The listing builds one solid part. Answer for the finished solid, in the listing's coordinates (mm). Face numbers are marked on the shaded views. A direction names the side the tool comes from. Coordinates: 2 decimals unless noted, no trailing zeros. Order: outer loops, then holes, each group sorted by start corner. A loop starts at its lowest first (then second) coordinate and runs counter-clockwise, first axis right, second up. Notation, with made-up numbers: (72.25, 16) -> (109.25, 16) arc R9 ccw to (109.25, 27) -> close; hole circle Ø2 at (36, 46.5). An arc over 180 degrees is marked (long way). Write item = value, one per line.
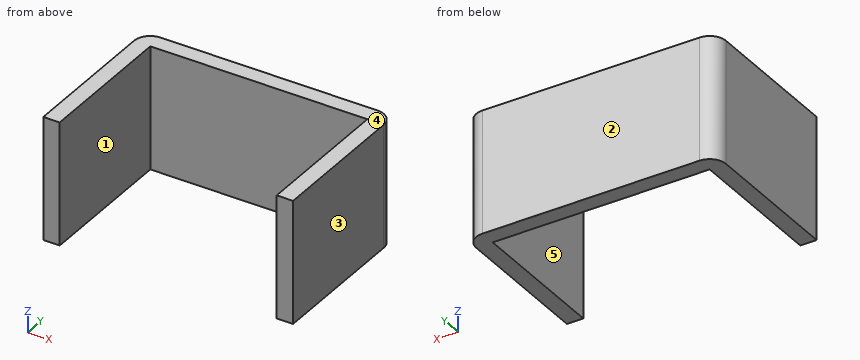
from build123d import *

# Parameters (mm, degrees)
BOSS_EXTRUDE1_DEPTH = 30


with BuildPart() as part:
    # Sketch1 → Boss-Extrude1 (new body)
    with BuildSketch(Plane.XY):
        with BuildLine():
            Line((0, 0), (0, 35))
            ThreePointArc((0, 35), (1.171572875, 37.828427125), (4, 39))
            Line((4, 39), (57, 39))
            ThreePointArc((57, 39), (59.828427125, 37.828427125), (61, 35))
            Line((61, 35), (61, 0))
            Line((61, 0), (57, 0))
            Line((57, 0), (57, 35))
            Line((57, 35), (4, 35))
            Line((4, 35), (4, 0))
            Line((4, 0), (0, 0))
        make_face()
    extrude(amount=BOSS_EXTRUDE1_DEPTH)


solid = part.part
Q1. Find the intervals of material crossed by line 1 along X through (y, z) = (11.5, 28.25); line 2 along Y through (x, z) = (56, 11.5); line 3 along Y through (x, z) = (3, 25), in increasing order.
The answers:
line_1 = 0 to 4, 57 to 61
line_2 = 35 to 39
line_3 = 0 to 38.87
Q2. Section C-C, the plane x = 43 is taken. Give the vertices of the cut face in (y, z), plus the area to 3 significant figures.
The answers:
outline = (35, 0) -> (39, 0) -> (39, 30) -> (35, 30) -> close
area = 120 mm2
Q3. A tool of negligible diameter and unlimited length cuts with its end or side. For the marked faces 1 and 2, from which of +Z, -Z, +X, -X, +Y, -Y can it reach the whole face along a straight path? Write none if from no direction.
The answers:
face_1 = +Z, -Z, -Y
face_2 = +Z, -Z, +X, -X, +Y
Q4. Section A-A, the plane y = 15 is taken. Give the vertices of the cut face in (x, z), plus the area to 3 significant figures.
The answers:
outline = (0, 0) -> (4, 0) -> (4, 30) -> (0, 30) -> close; (57, 0) -> (61, 0) -> (61, 30) -> (57, 30) -> close
area = 240 mm2
Q5. The mould has two halves that part along X. Classify the marked faces 3, 4 and 5: released by +X, released by -X, zero draft, split by the parting line, or undercut.
The answers:
face_3 = released by +X
face_4 = zero draft
face_5 = undercut
Q6. Section B-B, the plane z = 28 is taken. Give the vertices of the cut face in (x, y).
The answers:
outline = (0, 0) -> (4, 0) -> (4, 35) -> (57, 35) -> (57, 0) -> (61, 0) -> (61, 35) arc R4 ccw to (57, 39) -> (4, 39) arc R4 ccw to (0, 35) -> close
Q7. Each of these flat-tipped pins is pushed along its axis until it touches: pin 1 Ø1 at (x, z) = (32.5, 15) entering from -Y; pin 2 Ø6 at (x, z) = (6.5, 18) entering from -Y. Where does it stop, or does it pass through?
The answers:
pin_1 = 35
pin_2 = 0
